Verification items for the finished model (mm, model axes). Face numbers are marked on the shaded views. A direction names the side the tool comes from. Coordinates: 2 decimals unless noted, no trailing zeros. Write each loop counter-clockwise with the first axis right and the second up, starting at its lowest first coordinate (ties: lowest second). Pieces come first, ordered by that corner, then holes. Notation, with made-up numbers: (17, 86) -> (35, 86) arc R34 ccw to (35, 125) -> close; hole circle Ø3 at (-10.5, 53). An arc over 180 degrees is marked (long way). Use CSV: the item, a comma, the result in double quotes.
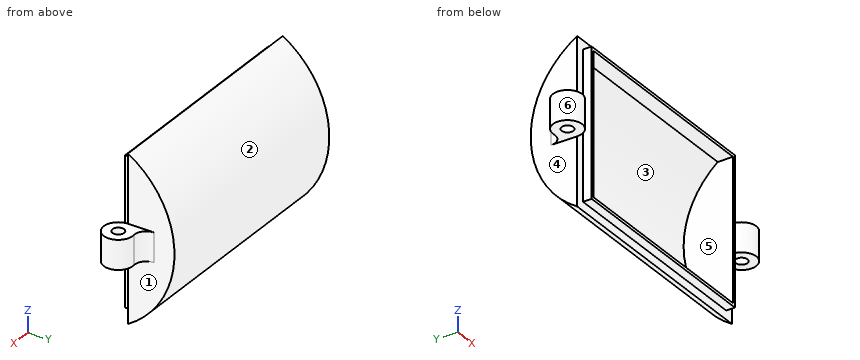
```python
from build123d import *

# Parameters (mm, degrees)
SKETCH2_R               = 16.5
BOSS_EXTRUDE1_DEPTH     = 40
SKETCH3_W               = 33
SKETCH3_H               = 25
CUT_EXTRUDE1_DEPTH      = 40
CUT_EXTRUDE2_REACH      = 45.174
CUT_EXTRUDE2_END_RADIUS = 15.5
SKETCH4_W               = 36
SKETCH4_H               = 24.284271248
SKETCH5_W               = 37
SKETCH5_H               = 25.284271248
SKETCH5_W_2             = 36
SKETCH5_H_2             = 24.284271248
BOSS_EXTRUDE2_DEPTH     = 1.5
SKETCH7_R               = 1
BOSS_EXTRUDE3_DEPTH     = 2.5


with BuildPart() as part:
    # Sketch2 → Boss-Extrude1 (new body)
    with BuildSketch(Plane(origin=(0, 0, 0), x_dir=(0, 0, -1), z_dir=(1, 0, 0))):
        Circle(SKETCH2_R)
    extrude(amount=BOSS_EXTRUDE1_DEPTH)

    # Sketch3 → Cut-Extrude1 (cut)
    with BuildSketch(Plane.ZY):
        with Locations((0, -4)):
            Rectangle(SKETCH3_W, SKETCH3_H)
    extrude(amount=-CUT_EXTRUDE1_DEPTH, mode=Mode.SUBTRACT)

    # Cut-Extrude2: up to this cylinder (the profile starts inside it)
    cut_extrude2_end = Plane(origin=(20, 0, 0), z_dir=(-1, 0, 0)) * Cylinder(CUT_EXTRUDE2_END_RADIUS, 122.348, mode=Mode.PRIVATE)
    # Sketch4 → Cut-Extrude2 (cut, up to the surface)
    with BuildSketch(Plane.XZ.offset(-8.5), mode=Mode.PRIVATE) as cut_extrude2_sk1:
        with Locations((20, 0)):
            Rectangle(SKETCH4_W, SKETCH4_H)
    cut_extrude2_tool1 = extrude(cut_extrude2_sk1.sketch, amount=-CUT_EXTRUDE2_REACH, mode=Mode.PRIVATE) & cut_extrude2_end
    add(cut_extrude2_tool1.solids().sort_by_distance((20, 8.5, 0))[0], mode=Mode.SUBTRACT)

    # Sketch5 → Boss-Extrude2 (add)
    with BuildSketch(Plane.XZ.offset(-8.5)):
        with Locations((20, 0)):
            Rectangle(SKETCH5_W, SKETCH5_H)
        with Locations((20, 0)):
            Rectangle(SKETCH5_W_2, SKETCH5_H_2, mode=Mode.SUBTRACT)
    extrude(amount=BOSS_EXTRUDE2_DEPTH)

    # Sketch7 → Boss-Extrude3 (add, symmetric)
    with BuildSketch(Plane.XY):
        with BuildLine():
            Line((40, 8.5), (40, 12.972135955))
            ThreePointArc((40, 12.972135955), (40.666666667, 11.48142397), (42.222222222, 10.984519975))
            ThreePointArc((42.222222222, 10.984519975), (44.363389981, 6.833333333), (40, 8.5))
        make_face()
        with Locations((42.5, 8.5)):
            Circle(SKETCH7_R, mode=Mode.SUBTRACT)
    boss_extrude3 = extrude(amount=BOSS_EXTRUDE3_DEPTH, both=True)

    # Mirror2: Boss-Extrude3 across plane
    add(boss_extrude3.mirror(Plane(origin=(20, 0, 0), x_dir=(0, 0, 1), z_dir=(1, 0, 0))))


solid = part.part
```
1) Mould release check, pull along X, two halves, no side actions. Record for the marked faces 1, 2, 3 and 4: released by +X, released by -X, zero draft, split by the parting line, or undercut.
Return value:
face 1,"released by +X"
face 2,"zero draft"
face 3,"undercut"
face 4,"released by -X"
2) Cross-section at B-B (x = 25). Record the boundary of the cut face in (y, z).
Return value:
outline,"(7, -12.64) -> (8.5, -12.64) -> (8.5, -14.14) arc R16.5 ccw to (8.5, 14.14) -> (8.5, 12.64) -> (7, 12.64) -> (7, 12.14) -> (9.63, 12.14) arc R15.5 cw to (9.63, -12.14) -> (7, -12.14) -> close"
3) Scan lines: L1, parallel to X at y = 7.5, z = 10.5; L2, parallel to Y at x = -2.5, z = -1.35; L3, parallel to Z at x = 31, y = 8.25. Record each from-to range of solid material in increasing order.
Return value:
L1,"1.5 to 2, 38 to 38.5"
L2,"6 to 7.5, 9.5 to 11"
L3,"-12.64 to -12.14, 12.14 to 12.64"
4) Set-up check for the marked faces 5 and 6: record each of +Z, -Z, +X, -X, +Y, -Y from which the full face is reachable in a straight line by a thin tool's end or side.
Return value:
face 5,"-Y"
face 6,"+Z, -Z"
5) Cross-section at A-A (y = 9). Record the boundary of the cut face in (x, z).
Return value:
outline,"(-4.95, -2.5) -> (-3.37, -2.5) -> (-3.37, 2.5) -> (-4.95, 2.5) -> close; (-1.63, -2.5) -> (0, -2.5) -> (0, -13.83) -> (40, -13.83) -> (40, -2.5) -> (41.63, -2.5) -> (41.63, 2.5) -> (40, 2.5) -> (40, 13.83) -> (0, 13.83) -> (0, 2.5) -> (-1.63, 2.5) -> close; (43.37, -2.5) -> (44.95, -2.5) -> (44.95, 2.5) -> (43.37, 2.5) -> close; hole (2, -12.14) -> (38, -12.14) -> (38, 12.14) -> (2, 12.14) -> close"
6) Cross-section at D-D (z = -9.25). Record the boundary of the cut face in (x, y), plus the area to 3 significant figures.
Return value:
outline,"(0, 8.5) -> (1.5, 8.5) -> (1.5, 7) -> (2, 7) -> (2, 12.44) -> (38, 12.44) -> (38, 7) -> (38.5, 7) -> (38.5, 8.5) -> (40, 8.5) -> (40, 13.66) -> (0, 13.66) -> close"
area,"66.3 mm2"
7) Gauge pin test, flat ends, axial feed: pin 1 (10 mm diameter, centred on x = 27.5, z = 8.5, fed in from +Y); pin 2 (1 mm diameter, centred on x = 14, z = -10, fed in from +Y); pin 3 (1.6 mm diameter, centred on x = 18, y = 7.5, fed in from +Z). Record the tip position at first contact, or that the pin passes through.
Return value:
pin 1,"y = 16.12"
pin 2,"y = 13.49"
pin 3,"z = 12.64"
8) Cross-section at C-C (z = -1). Record the boundary of the cut face in (x, y).
Return value:
outline,"(-2.22, 10.98) arc R2.5 ccw (long way) to (0, 8.5) -> (1.5, 8.5) -> (1.5, 7) -> (2, 7) -> (2, 15.47) -> (38, 15.47) -> (38, 7) -> (38.5, 7) -> (38.5, 8.5) -> (40, 8.5) arc R2.5 ccw (long way) to (42.22, 10.98) arc R2 cw to (40, 12.97) -> (40, 16.47) -> (0, 16.47) -> (0, 12.97) arc R2 cw to start; hole circle Ø2 at (-2.5, 8.5); hole circle Ø2 at (42.5, 8.5)"
